Can you work these out from the model? Positions are in its coordinate system, mm. Give positions to 0.01 mm unless a question says otherwise; leave off trailing zeros. Order: outer loops, then holes, each group sorted by start corner. A loop starts at its lowest first (then second) coordinate and runs counter-clockwise, first axis right, second up. Notation, with made-up numbers: M 72.5,-12.75 L 119.5,-12.75 A22 ccw 119.5,9.25 Z; hole C 30.5,58.25 d6. An arc over 180 degrees is marked long. Use one line per item in the form item = value. Start each with the question number.
1. I want a section at C-C, the plane y = 6.35. List the corners of the cut face in (x, z) for me, and give its area (3 significant figures).
2. I want a section at D-D, the plane y = 34.5. List the corners of the cut face in (x, z) for me.
3. I want a section at A-A, the plane x = 0. List the corners of the cut face in (y, z) for me.
4. I want a section at B-B, the plane z = -5. List the corners of the cut face in (x, y) for me.
5. Will these pins go through, and if not, where does the flat tip stop? P1, Ø1.9, axis at y = 42.5, z = -3, coming from the +X side; P2, Ø17.5, axis at x = 0, y = 6.35, coming from the -Z side.
6. I need wall thicknesses on L1, parallel to Y at x = 0, z = -3; L2, parallel to X at y = 62.5, z = -2.75; L3, parallel to Y at x = 18.5, z = -1. Which ranges of each line are inside material? Lowest first, please.
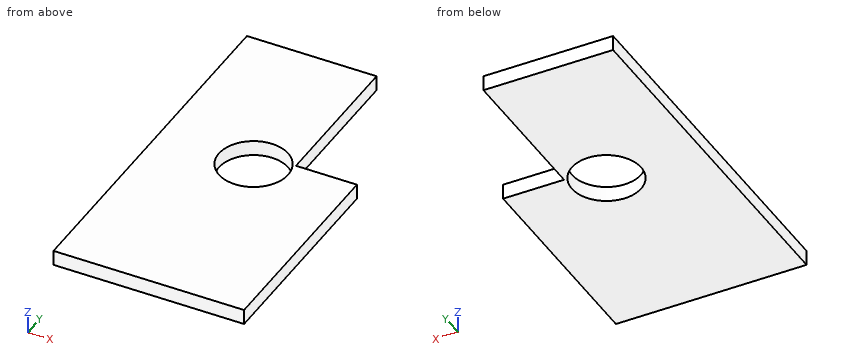
Autodesk Inventor part; units mm, degrees
ref_plane "YZ Plane" through (0, 0, 0) normal (1, 0, 0) x (0, 1, 0)
ref_plane "XZ Plane" through (0, 0, 0) normal (0, 1, 0) x (-1, 0, 0)
ref_plane "XY Plane" through (0, 0, 0) normal (0, 0, 1) x (1, 0, 0)
sketch "Sketch1" plane through (0, 0, 0) normal (0, 0, 1) x (1, 0, 0)
  line L0 (-39.6875, -76.2) -> (39.6875, -76.2)
  line L1 (39.6875, -76.2) -> (39.6875, 76.2)
  line L2 (39.6875, 76.2) -> (-39.6875, 76.2)
  line L3 (-39.6875, 76.2) -> (-39.6875, -76.2)
  line L4 (-39.6875, -76.2) -> (39.6875, 76.2) construction
  line L5 (39.6875, -76.2) -> (-39.6875, 76.2) construction
  point P0 (0, 0)
  dimension "d0" = 79.375
  dimension "d1" = 152.4
extrude "Extrusion1" add sketch "Sketch1" against normal blind 6.35
sketch "Sketch2" plane through (0, 0, 0) normal (0, 0, 1) x (1, 0, 0)
  circle A0 centre (0, 6.35) radius 14.4145
  line L0 (39.6875, 76.2) -> (-39.6875, 76.2)
  point P0 (0, 0)
  dimension "bearingDiameter" = 28.829
  dimension "d5" = 69.85
extrude "Extrusion2" cut sketch "Sketch2" against normal through all
sketch "Sketch8" plane through (0, 0, 0) normal (0, 0, 1) x (1, 0, 0)
  line L0 (-39.6875, 76.2) -> (39.6875, 76.2)
  line L1 (39.6875, 76.2) -> (14.2875, 76.2)
  line L2 (14.2875, 76.2) -> (14.2875, 12.7)
  line L3 (14.2875, 12.7) -> (39.6875, 12.7)
  line L4 (39.6875, 12.7) -> (39.6875, 76.2)
  point P0 (0, 0)
  dimension "d43" = 25.4
  dimension "d44" = 63.5
extrude "Extrusion3" cut sketch "Sketch8" against normal through all
properties part number "plateForHangingMechanism" material "Aluminum 6061"
Check result:
q1.outline = M -39.69,-6.35 L -14.41,-6.35 L -14.41,0 L -39.69,0 Z; M 14.41,-6.35 L 39.69,-6.35 L 39.69,0 L 14.41,0 Z
q1.area = 321 mm2
q2.outline = M -39.69,-6.35 L 14.29,-6.35 L 14.29,0 L -39.69,0 Z
q3.outline = M -76.2,-6.35 L -8.06,-6.35 L -8.06,0 L -76.2,0 Z; M 20.76,-6.35 L 76.2,-6.35 L 76.2,0 L 20.76,0 Z
q4.outline = M -39.69,-76.2 L 39.69,-76.2 L 39.69,12.7 L 14.29,12.7 L 14.29,76.2 L -39.69,76.2 Z; hole C 0,6.35 d28.83
q5.P1 = 14.29
q5.P2 = through
q6.L1 = -76.2 to -8.06, 20.76 to 76.2
q6.L2 = -39.69 to 14.29
q6.L3 = -76.2 to 12.7
